```python
from build123d import *

# Parameters (mm, degrees)
SKETCH_10_R                   = 10
SM_BASE_FLANGE_3_DEPTH        = 2
SM_EDGE_FLANGE_6_DEPTH        = 230
SM_EDGE_FLANGE_6_BEND_DEPTH   = 230
SM_EDGE_FLANGE_6_BEND_2_DEPTH = 230
CUT_EXTRUDE_4_REACH           = 363.137
SKETCH_47_R                   = 2
CUT_EXTRUDE_6_REACH           = 263.424
SKETCH_50_R                   = 2
CUT_EXTRUDE_7_REACH           = 351.772
SKETCH_51_R                   = 2
CUT_EXTRUDE_8_REACH           = 349.61
SKETCH_52_R                   = 14
SKETCH_53_R                   = 1.5
CUT_EXTRUDE_9_DEPTH           = 10


# Sheet-metal steps are written as plain solids
with BuildPart() as part:
    # Эскиз10 → Базовая кромка3 (new body)
    with BuildSketch(Plane.XY):
        Polygon((0, 0), (-21, 36.373066959), (94, 235.558909829), (136, 235.558909829), (251, 36.373066959), (230, 0), align=None)
        with Locations((171.849364905, 123.465988394)):
            Circle(SKETCH_10_R, mode=Mode.SUBTRACT)
    extrude(amount=-SM_BASE_FLANGE_3_DEPTH)

    # Ребро-кромка6 section (across the edge) → Ребро-кромка6 (add)
    with BuildSketch(Plane(origin=(-21.866025404, 36.873066959, -2), x_dir=(0.8660254037844436, -0.4999999999999914, -3.4914813388431334e-15), z_dir=(0.4999999999999914, 0.8660254037844436, 0))):
        with BuildLine():
            Line((-2, 1), (-2, 18))
            Line((-2, 18), (0, 18))
            Line((0, 18), (0, 1))
            ThreePointArc((0, 1), (0.292893219, 0.292893219), (1, 0))
            Line((1, 0), (1, -2))
            ThreePointArc((1, -2), (-1.121320344, -1.121320344), (-2, 1))
        make_face()
    extrude(amount=SM_EDGE_FLANGE_6_DEPTH)

    # Ребро-кромка6 section 2 (across the edge) → Ребро-кромка6 bend (add)
    with BuildSketch(Plane(origin=(136.866025404, 236.058909829, -2), x_dir=(-0.8660254037844363, -0.5000000000000041, -3.4914813388431334e-15), z_dir=(0.5000000000000041, -0.8660254037844363, 0))):
        with BuildLine():
            Line((-2, 1), (-2, 18))
            Line((-2, 18), (0, 18))
            Line((0, 18), (0, 1))
            ThreePointArc((0, 1), (0.292893219, 0.292893219), (1, 0))
            Line((1, 0), (1, -2))
            ThreePointArc((1, -2), (-1.121320344, -1.121320344), (-2, 1))
        make_face()
    extrude(amount=SM_EDGE_FLANGE_6_BEND_DEPTH)

    # Ребро-кромка6 section 3 (across the edge) → Ребро-кромка6 bend 2 (add)
    with BuildSketch(Plane(origin=(230, -1, -2), x_dir=(0, 1, 0), z_dir=(-1, 0, 0))):
        with BuildLine():
            Line((-2, 1), (-2, 18))
            Line((-2, 18), (0, 18))
            Line((0, 18), (0, 1))
            ThreePointArc((0, 1), (0.292893219, 0.292893219), (1, 0))
            Line((1, 0), (1, -2))
            ThreePointArc((1, -2), (-1.121320344, -1.121320344), (-2, 1))
        make_face()
    extrude(amount=SM_EDGE_FLANGE_6_BEND_2_DEPTH)

    # Эскиз47 → Вырез-Вытянуть4 (cut, up to next)
    with BuildSketch(Plane(origin=(-34.098076211, 19.686533479, 0), x_dir=(0, 0, 1), z_dir=(-0.866025403784443, 0.4999999999999925, 3.788649256556814e-15)), mode=Mode.PRIVATE) as cut_extrude_4_sk1:
        with Locations(Location((-11.5, 29, 0), (0, 0, 270))):
            Circle(SKETCH_47_R)
    cut_extrude_4_tool1 = extrude(cut_extrude_4_sk1.sketch, amount=-CUT_EXTRUDE_4_REACH, mode=Mode.PRIVATE) & part.part
    # Эскиз47 → Вырез-Вытянуть4 (cut, up to next)
    with BuildSketch(Plane(origin=(-34.098076211, 19.686533479, 0), x_dir=(0, 0, 1), z_dir=(-0.866025403784443, 0.4999999999999925, 3.788649256556814e-15)), mode=Mode.PRIVATE) as cut_extrude_4_sk2:
        with Locations(Location((-11.5, 39, 0), (0, 0, 270))):
            Circle(SKETCH_47_R)
    cut_extrude_4_tool2 = extrude(cut_extrude_4_sk2.sketch, amount=-CUT_EXTRUDE_4_REACH, mode=Mode.PRIVATE) & part.part
    # Эскиз47 → Вырез-Вытянуть4 (cut, up to next)
    with BuildSketch(Plane(origin=(-34.098076211, 19.686533479, 0), x_dir=(0, 0, 1), z_dir=(-0.866025403784443, 0.4999999999999925, 3.788649256556814e-15)), mode=Mode.PRIVATE) as cut_extrude_4_sk3:
        with Locations(Location((-11.5, 233, 0), (0, 0, 270))):
            Circle(SKETCH_47_R)
    cut_extrude_4_tool3 = extrude(cut_extrude_4_sk3.sketch, amount=-CUT_EXTRUDE_4_REACH, mode=Mode.PRIVATE) & part.part
    # Эскиз47 → Вырез-Вытянуть4 (cut, up to next)
    with BuildSketch(Plane(origin=(-34.098076211, 19.686533479, 0), x_dir=(0, 0, 1), z_dir=(-0.866025403784443, 0.4999999999999925, 3.788649256556814e-15)), mode=Mode.PRIVATE) as cut_extrude_4_sk4:
        with Locations(Location((-11.5, 243, 0), (0, 0, 270))):
            Circle(SKETCH_47_R)
    cut_extrude_4_tool4 = extrude(cut_extrude_4_sk4.sketch, amount=-CUT_EXTRUDE_4_REACH, mode=Mode.PRIVATE) & part.part
    add(cut_extrude_4_tool1.solids().sort_by_distance((-19.598076, 44.80127, -11.5))[0], mode=Mode.SUBTRACT)
    add(cut_extrude_4_tool2.solids().sort_by_distance((-14.598076, 53.461524, -11.5))[0], mode=Mode.SUBTRACT)
    add(cut_extrude_4_tool3.solids().sort_by_distance((82.401924, 221.470453, -11.5))[0], mode=Mode.SUBTRACT)
    add(cut_extrude_4_tool4.solids().sort_by_distance((87.401924, 230.130707, -11.5))[0], mode=Mode.SUBTRACT)

    # Эскиз50 → Вырез-Вытянуть6 (cut, up to next)
    with BuildSketch(Plane(origin=(206.598076211, 119.279454915, 0), x_dir=(0, 0, -1), z_dir=(0.866025403784436, 0.5000000000000047, 3.0623287353932815e-15)), mode=Mode.PRIVATE) as cut_extrude_6_sk1:
        with Locations(Location((11.5, -86, 0), (0, 0, 90))):
            Circle(SKETCH_50_R)
    cut_extrude_6_tool1 = extrude(cut_extrude_6_sk1.sketch, amount=-CUT_EXTRUDE_6_REACH, mode=Mode.PRIVATE) & part.part
    # Эскиз50 → Вырез-Вытянуть6 (cut, up to next)
    with BuildSketch(Plane(origin=(206.598076211, 119.279454915, 0), x_dir=(0, 0, -1), z_dir=(0.866025403784436, 0.5000000000000047, 3.0623287353932815e-15)), mode=Mode.PRIVATE) as cut_extrude_6_sk2:
        with Locations(Location((11.5, -76, 0), (0, 0, 90))):
            Circle(SKETCH_50_R)
    cut_extrude_6_tool2 = extrude(cut_extrude_6_sk2.sketch, amount=-CUT_EXTRUDE_6_REACH, mode=Mode.PRIVATE) & part.part
    # Эскиз50 → Вырез-Вытянуть6 (cut, up to next)
    with BuildSketch(Plane(origin=(206.598076211, 119.279454915, 0), x_dir=(0, 0, -1), z_dir=(0.866025403784436, 0.5000000000000047, 3.0623287353932815e-15)), mode=Mode.PRIVATE) as cut_extrude_6_sk3:
        with Locations(Location((11.5, 118, 0), (0, 0, 90))):
            Circle(SKETCH_50_R)
    cut_extrude_6_tool3 = extrude(cut_extrude_6_sk3.sketch, amount=-CUT_EXTRUDE_6_REACH, mode=Mode.PRIVATE) & part.part
    # Эскиз50 → Вырез-Вытянуть6 (cut, up to next)
    with BuildSketch(Plane(origin=(206.598076211, 119.279454915, 0), x_dir=(0, 0, -1), z_dir=(0.866025403784436, 0.5000000000000047, 3.0623287353932815e-15)), mode=Mode.PRIVATE) as cut_extrude_6_sk4:
        with Locations(Location((11.5, 128, 0), (0, 0, 90))):
            Circle(SKETCH_50_R)
    cut_extrude_6_tool4 = extrude(cut_extrude_6_sk4.sketch, amount=-CUT_EXTRUDE_6_REACH, mode=Mode.PRIVATE) & part.part
    add(cut_extrude_6_tool1.solids().sort_by_distance((249.598076, 44.80127, -11.5))[0], mode=Mode.SUBTRACT)
    add(cut_extrude_6_tool2.solids().sort_by_distance((244.598076, 53.461524, -11.5))[0], mode=Mode.SUBTRACT)
    add(cut_extrude_6_tool3.solids().sort_by_distance((147.598076, 221.470453, -11.5))[0], mode=Mode.SUBTRACT)
    add(cut_extrude_6_tool4.solids().sort_by_distance((142.598076, 230.130707, -11.5))[0], mode=Mode.SUBTRACT)

    # Эскиз51 → Вырез-Вытянуть7 (cut, up to next)
    with BuildSketch(Plane.XZ.offset(3), mode=Mode.PRIVATE) as cut_extrude_7_sk1:
        with Locations(Location((222, -11.5, 0), (0, 0, 270))):
            Circle(SKETCH_51_R)
    cut_extrude_7_tool1 = extrude(cut_extrude_7_sk1.sketch, amount=-CUT_EXTRUDE_7_REACH, mode=Mode.PRIVATE) & part.part
    # Эскиз51 → Вырез-Вытянуть7 (cut, up to next)
    with BuildSketch(Plane.XZ.offset(3), mode=Mode.PRIVATE) as cut_extrude_7_sk2:
        with Locations(Location((212, -11.5, 0), (0, 0, 270))):
            Circle(SKETCH_51_R)
    cut_extrude_7_tool2 = extrude(cut_extrude_7_sk2.sketch, amount=-CUT_EXTRUDE_7_REACH, mode=Mode.PRIVATE) & part.part
    # Эскиз51 → Вырез-Вытянуть7 (cut, up to next)
    with BuildSketch(Plane.XZ.offset(3), mode=Mode.PRIVATE) as cut_extrude_7_sk3:
        with Locations(Location((18, -11.5, 0), (0, 0, 270))):
            Circle(SKETCH_51_R)
    cut_extrude_7_tool3 = extrude(cut_extrude_7_sk3.sketch, amount=-CUT_EXTRUDE_7_REACH, mode=Mode.PRIVATE) & part.part
    # Эскиз51 → Вырез-Вытянуть7 (cut, up to next)
    with BuildSketch(Plane.XZ.offset(3), mode=Mode.PRIVATE) as cut_extrude_7_sk4:
        with Locations(Location((8, -11.5, 0), (0, 0, 270))):
            Circle(SKETCH_51_R)
    cut_extrude_7_tool4 = extrude(cut_extrude_7_sk4.sketch, amount=-CUT_EXTRUDE_7_REACH, mode=Mode.PRIVATE) & part.part
    add(cut_extrude_7_tool1.solids().sort_by_distance((222, -3, -11.5))[0], mode=Mode.SUBTRACT)
    add(cut_extrude_7_tool2.solids().sort_by_distance((212, -3, -11.5))[0], mode=Mode.SUBTRACT)
    add(cut_extrude_7_tool3.solids().sort_by_distance((18, -3, -11.5))[0], mode=Mode.SUBTRACT)
    add(cut_extrude_7_tool4.solids().sort_by_distance((8, -3, -11.5))[0], mode=Mode.SUBTRACT)

    # Эскиз52 → Вырез-Вытянуть8 (cut, up to next)
    with BuildSketch(Plane(origin=(0, 0, -2), x_dir=(-1, 0, 0), z_dir=(0, 0, -1)), mode=Mode.PRIVATE) as cut_extrude_8_sk1:
        with Locations((-115, 90.643992263)):
            Circle(SKETCH_52_R)
    cut_extrude_8_tool1 = extrude(cut_extrude_8_sk1.sketch, amount=-CUT_EXTRUDE_8_REACH, mode=Mode.PRIVATE) & part.part
    add(cut_extrude_8_tool1.solids().sort_by_distance((115, 90.643992, -2))[0], mode=Mode.SUBTRACT)

    # Эскиз53 → Вырез-Вытянуть9 (cut)
    with BuildSketch(Plane(origin=(0, 0, -2), x_dir=(-1, 0, 0), z_dir=(0, 0, -1))):
        with Locations((-40.121778265, 70.507041555)):
            Circle(SKETCH_53_R)
        with Locations((-22.801270189, 60.507041555)):
            Circle(SKETCH_53_R)
        with Locations((-60.121778265, 35.866025404)):
            Circle(SKETCH_53_R)
        with Locations((-42.801270189, 25.866025404)):
            Circle(SKETCH_53_R)
        with Locations((-95, 185.558909829)):
            Circle(SKETCH_53_R)
        with Locations((-95, 165.558909829)):
            Circle(SKETCH_53_R)
        with Locations((-135, 185.558909829)):
            Circle(SKETCH_53_R)
        with Locations((-135, 165.558909829)):
            Circle(SKETCH_53_R)
        with Locations((-207.198729811, 60.507041555)):
            Circle(SKETCH_53_R)
        with Locations((-189.878221735, 70.507041555)):
            Circle(SKETCH_53_R)
        with Locations((-187.198729811, 25.866025404)):
            Circle(SKETCH_53_R)
        with Locations((-169.878221735, 35.866025404)):
            Circle(SKETCH_53_R)
    extrude(amount=-CUT_EXTRUDE_9_DEPTH, mode=Mode.SUBTRACT)


solid = part.part
```
Work out the finished part from the listing and answer in its coordinate system (mm). A direction names the side the tool comes from. Give positions to 0.01 mm unless a question says otherwise; leave off trailing zeros. Loops run counter-clockwise (first coordinate to the right, second up) from the corner with the lowest first, then second, coordinate; pieces in that order, holes last. Notation, with made-up numbers: (54.5, 75.5) -> (69.5, 75.5) arc R19 ccw to (69.5, 107.5) -> close; hole circle Ø1 at (-34, 69.5). An arc over 180 degrees is marked (long way). One line per question, with ' | ' between items. Start each with the question number.
1) Determine the mould class of faces 3 (the face through (117, -1, -12)), 4 (the face through (-10.35, 17.93, -0.99)), 5 (the face through (34.83, 135.07, -11.62)) for opening direction X: +X half, -X half, draft (parallel to the pull), parting line (faces both ways), or undercut.
2) Section B-B, the plane x = 115 is taken. Determine the outline of the cut face in (y, z).
3) Each of these flat-tipped pins is pushed along its axis until it touches: pin 1 (12 mm diameter, centred on y = 71, z = -13, fed in from -X); pin 2 (4 mm diameter, centred on x = 40.12, y = 70.51, fed in from -Z); pin 3 (8.5 mm diameter, centred on x = 94.5, z = -12.5, fed in from +Y); pin 4 (12 mm diameter, centred on x = 64.5, y = 175.5, fed in from -Z). Where does it stop, or does it pass through?
4) For faces 1 (the face through (240.647, 18.441, -0.986)), 2 (the face through (117, 67, -2)), determine the directions among +Z, -Z, +X, -X, +Y, -Y from which every point of the face is accessible in a straight line to the end or side of a thin tool.
5) Section A-A, the plane z = -17 is taken. Determine the outline of the cut face in (x, y), then the cut area to 3 significant figures.
6) Straight lines are drawn through the part: L1, parallel to Z at x = 216, y = 47; L2, parallel to Y at x = 92, z = -14.25; L3, parallel to X at y = 138, z = -14.5. For each, find the intervals that lie inside material, in ascending order.
7) Section C-C, the plane y = 21 is taken. Determine the outline of the cut face in (x, z).
Resolved:
1) face 3: draft | face 4: -X half | face 5: undercut
2) outline: (-3, -20) -> (-1, -20) -> (-1, -3) arc R1 cw to (0, -2) -> (76.64, -2) -> (76.64, 0) -> (0, 0) arc R3 ccw to (-3, -3) -> close; (104.64, -2) -> (235.56, -2) -> (235.56, 0) -> (104.64, 0) -> close
3) pin 1: x = -7.94 | pin 2: z = -2 | pin 3: y = 237.06 | pin 4: z = -20
4) face 1: +Z, -Z, +X, -Y | face 2: -Z
5) outline: (-23.6, 37.87) -> (-21.87, 36.87) -> (93.13, 236.06) -> (91.4, 237.06) -> close; (0, -3) -> (230, -3) -> (230, -1) -> (0, -1) -> close; (136.87, 236.06) -> (251.87, 36.87) -> (253.6, 37.87) -> (138.6, 237.06) -> close | area: 1,380 mm2
6) L1: -2 to 0 | L2: -3 to -1, 234.09 to 236.71 | L3: 34.21 to 36.52, 193.48 to 195.79
7) outline: (-12.12, -2) -> (242.12, -2) -> (242.12, 0) -> (-12.12, 0) -> close
